The model under review builds one solid part; all positions refer to its coordinate system, in mm. Give positions to 0.01 mm unless a question says otherwise; leave off trailing zeros. Order: outer loops, then holes, each group sorted by start corner. A loop starts at its lowest first (then second) coordinate and runs counter-clockwise, first axis right, second up. Notation, with made-up numbers: (61.25, 16.5) - (91.25, 16.5) arc R28 ccw to (91.25, 43.5) - close; hole circle Ø4 at (33.5, -31). An arc over 180 degrees is marked (long way). Write item = value, one per line. Start each with the question number.
1. We need section A-A, the plane z = 673.1. Give the boundary of the cut face in (x, y) (1 decimal).
2. Wall thickness on probe 1 along Y at (x, z) = (1.05, 571.5); probe 2 along Y at (x, z) = (1, 203.2) (3 decimals); probe 3 along Y at (x, z) = (2.1, 153): over which ranges is each line inside the solid? List them lowest first.
3. We need section B-B, the plane x = 2.3. State how many separate pieces and enclosed holes the cut face has, and give its area (3 significant figures).
from build123d import *

# Parameters (mm, degrees)
SKETCH1_R           = 7.9629
SKETCH1_R_2         = 3.3782
SKETCH1_R_3         = 2.5527
SKETCH1_R_4         = 14.2875
SKETCH1_R_5         = 1.89865
SKETCH1_R_6         = 3.1496
SKETCH1_R_7         = 3.175
BOSS_EXTRUDE1_DEPTH = 3.175


with BuildPart() as part:
    # Sketch1 → Boss-Extrude1 (new body)
    with BuildSketch(Plane(origin=(0, 0, 0), x_dir=(0, 0, -1), z_dir=(1, 0, 0))):
        with BuildLine():
            Line((-12.7, 0), (-698.5, 0))
            ThreePointArc((-698.5, 0), (-707.480256121, 3.719743879), (-711.2, 12.7))
            Line((-711.2, 12.7), (-711.2, 38.1))
            ThreePointArc((-711.2, 38.1), (-707.480256121, 47.080256121), (-698.5, 50.8))
            Line((-698.5, 50.8), (-12.7, 50.8))
            ThreePointArc((-12.7, 50.8), (-3.719743879, 47.080256121), (0, 38.1))
            Line((0, 38.1), (0, 12.7))
            ThreePointArc((0, 12.7), (-3.719743879, 3.719743879), (-12.7, 0))
        make_face()
        with Locations((-50.8, 25.4)):
            Circle(SKETCH1_R, mode=Mode.SUBTRACT)
        with Locations((-28.575, 25.4)):
            Circle(SKETCH1_R_2, mode=Mode.SUBTRACT)
        with Locations((-215.9, 44.45)):
            Circle(SKETCH1_R_3, mode=Mode.SUBTRACT)
        with Locations((-190.5, 44.45)):
            Circle(SKETCH1_R_3, mode=Mode.SUBTRACT)
        with Locations((-190.5, 6.35)):
            Circle(SKETCH1_R_3, mode=Mode.SUBTRACT)
        with Locations((-215.9, 6.35)):
            Circle(SKETCH1_R_3, mode=Mode.SUBTRACT)
        with Locations((-73.025, 25.4)):
            Circle(SKETCH1_R_2, mode=Mode.SUBTRACT)
        with Locations((-673.1, 25.4)):
            Circle(SKETCH1_R_4, mode=Mode.SUBTRACT)
        with Locations((-571.5, 44.45)):
            Circle(SKETCH1_R_3, mode=Mode.SUBTRACT)
        with Locations((-546.1, 44.45)):
            Circle(SKETCH1_R_3, mode=Mode.SUBTRACT)
        with Locations((-12.7, 38.1)):
            Circle(SKETCH1_R_5, mode=Mode.SUBTRACT)
        with Locations((-12.7, 12.7)):
            Circle(SKETCH1_R_5, mode=Mode.SUBTRACT)
        with Locations((-546.1, 6.35)):
            Circle(SKETCH1_R_3, mode=Mode.SUBTRACT)
        with Locations((-571.5, 6.35)):
            Circle(SKETCH1_R_3, mode=Mode.SUBTRACT)
        with Locations((-558.8, 12.7)):
            Circle(SKETCH1_R_6, mode=Mode.SUBTRACT)
        with Locations((-203.2, 38.1)):
            Circle(SKETCH1_R_7, mode=Mode.SUBTRACT)
        with Locations((-698.5, 38.1)):
            Circle(SKETCH1_R_5, mode=Mode.SUBTRACT)
        with Locations((-698.5, 12.7)):
            Circle(SKETCH1_R_5, mode=Mode.SUBTRACT)
        with Locations((-558.8, 38.1)):
            Circle(SKETCH1_R_5, mode=Mode.SUBTRACT)
        with Locations((-203.2, 12.7)):
            Circle(SKETCH1_R_5, mode=Mode.SUBTRACT)
        with Locations((-381, 25.4)):
            Circle(SKETCH1_R_5, mode=Mode.SUBTRACT)
        Polygon((-228.6, 38.1), (-228.6, 12.7), (-273.05, 12.7), align=None, mode=Mode.SUBTRACT)
        Polygon((-635, 38.1), (-635, 12.7), (-596.9, 12.7), align=None, mode=Mode.SUBTRACT)
        Polygon((-622.3, 38.1), (-584.2, 38.1), (-584.2, 12.7), align=None, mode=Mode.SUBTRACT)
        Polygon((-533.4, 38.1), (-533.4, 12.7), (-488.95, 12.7), align=None, mode=Mode.SUBTRACT)
        Polygon((-406.4, 38.1), (-406.4, 12.7), (-450.85, 38.1), align=None, mode=Mode.SUBTRACT)
        Polygon((-419.1, 12.7), (-463.55, 38.1), (-463.55, 12.7), align=None, mode=Mode.SUBTRACT)
        Polygon((-476.25, 12.7), (-476.25, 38.1), (-520.7, 38.1), align=None, mode=Mode.SUBTRACT)
        Polygon((-241.3, 38.1), (-285.75, 12.7), (-285.75, 38.1), align=None, mode=Mode.SUBTRACT)
        Polygon((-298.45, 38.1), (-298.45, 12.7), (-342.9, 12.7), align=None, mode=Mode.SUBTRACT)
        Polygon((-355.6, 38.1), (-355.6, 12.7), (-311.15, 38.1), align=None, mode=Mode.SUBTRACT)
        Polygon((-177.8, 38.1), (-177.8, 12.7), (-111.125, 38.1), align=None, mode=Mode.SUBTRACT)
        Polygon((-85.725, 38.1), (-85.725, 12.7), (-152.4, 12.7), align=None, mode=Mode.SUBTRACT)
    extrude(amount=BOSS_EXTRUDE1_DEPTH)


solid = part.part
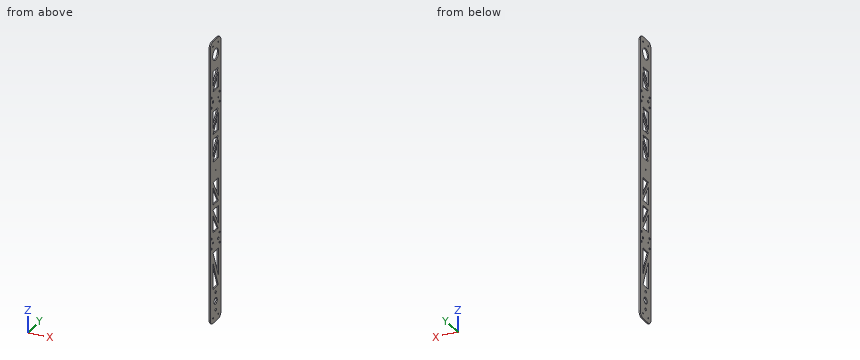
Model answer:
q1.outline = (0, 0) - (3.2, 0) - (3.2, 11.1) - (0, 11.1) - close; (0, 39.7) - (3.2, 39.7) - (3.2, 50.8) - (0, 50.8) - close
q2.probe_1 = 0 to 3.8, 8.9 to 41.9, 47 to 50.8
q2.probe_2 = 0 to 10.801, 14.599 to 34.925, 41.275 to 50.8
q2.probe_3 = 0 to 22.15, 38.1 to 50.8
q3.separate_pieces = 1
q3.enclosed_holes = 33
q3.area = 27,600 mm2
